from build123d import *

# Parameters (mm, degrees)
EXTRUDE_1_DEPTH     = 50
SKETCH_2_R          = 11.05
CUT_EXTRUDE_1_DEPTH = 88.76388779
CHAMFER_1_SIZE      = 5
SKETCH_3_R          = 1.75
CUT_EXTRUDE_2_DEPTH = 88.76388779
EXTRUDE_3_DEPTH     = 3
EXTRUDE_START       = -3
EXTRUDE_4_DEPTH     = 3
CUT_EXTRUDE_3_DEPTH = 88.832226432


with BuildPart() as part:
    # 草图1 → 凸台-拉伸1 (new body)
    with BuildSketch(Plane(origin=(0, 0, 0), x_dir=(0, 0, -1), z_dir=(1, 0, 0))):
        Polygon((0, 0), (3, 0), (3, -48.5), (53.5, -48.5), (53.5, -51.5), (0, -51.5), align=None)
    extrude(amount=EXTRUDE_1_DEPTH)

    # 草图2 → 切除-拉伸1 (cut, through all)
    with BuildSketch(Plane(origin=(0, 0, -3), x_dir=(-1, 0, 0), z_dir=(0, 0, -1))):
        with Locations(Location((-25, -21, 0), (0, 0, 90))):
            Circle(SKETCH_2_R)
    extrude(amount=-CUT_EXTRUDE_1_DEPTH, mode=Mode.SUBTRACT)

    # 倒角1
    chamfer_1_edges = [part.edges().sort_by_distance(p)[0] for p in [
        (50, -50, -53.5),
        (50, 0, -1.5),
        (0, 0, -1.5),
        (0, -50, -53.5),
    ]]
    chamfer(chamfer_1_edges, length=CHAMFER_1_SIZE)

    # 草图3 → 切除-拉伸2 (cut, through all)
    with BuildSketch(Plane(origin=(0, 0, -3), x_dir=(-1, 0, 0), z_dir=(0, 0, -1))):
        with Locations(Location((-40.5, -5.5, 0), (0, 0, 90))):
            Circle(SKETCH_3_R)
        with Locations(Location((-9.5, -5.5, 0), (0, 0, 90))):
            Circle(SKETCH_3_R)
        with Locations(Location((-9.5, -36.5, 0), (0, 0, 90))):
            Circle(SKETCH_3_R)
        with Locations(Location((-40.5, -36.5, 0), (0, 0, 90))):
            Circle(SKETCH_3_R)
    extrude(amount=-CUT_EXTRUDE_2_DEPTH, mode=Mode.SUBTRACT)

    # 草图4 → 凸台-拉伸3 (add)
    with BuildSketch(Plane(origin=(50, 0, 0), x_dir=(0, 0, -1), z_dir=(1, 0, 0))):
        with BuildLine():
            Line((3, -28.5), (16, -48.5))
            Line((16, -48.5), (5, -48.5))
            ThreePointArc((5, -48.5), (3.585786438, -47.914213562), (3, -46.5))
            Line((3, -46.5), (3, -28.5))
        make_face()
    extrude(amount=-EXTRUDE_3_DEPTH)

    # 草图5 → 凸台-拉伸4 (add)
    with BuildSketch(Plane.ZY.offset(EXTRUDE_START)):
        with BuildLine():
            Line((-5, -48.5), (-16, -48.5))
            Line((-16, -48.5), (-3, -28.5))
            Line((-3, -28.5), (-3, -46.5))
            ThreePointArc((-3, -46.5), (-3.585786438, -47.914213562), (-5, -48.5))
        make_face()
    extrude(amount=EXTRUDE_4_DEPTH)

    # 草图6 → 切除-拉伸3 (cut, through all)
    with BuildSketch(Plane(origin=(0, -48.5, 0), x_dir=(1, 0, 0), z_dir=(0, 1, 0))):
        with BuildLine():
            Line((12.1, 42.5), (12.1, 12.5))
            ThreePointArc((12.1, 12.5), (10, 10.4), (7.9, 12.5))
            Line((7.9, 12.5), (7.9, 42.5))
            ThreePointArc((7.9, 42.5), (10, 44.6), (12.1, 42.5))
        make_face()
        with BuildLine():
            Line((42.1, 42.5), (42.1, 12.5))
            ThreePointArc((42.1, 12.5), (40, 10.4), (37.9, 12.5))
            Line((37.9, 12.5), (37.9, 42.5))
            ThreePointArc((37.9, 42.5), (40, 44.6), (42.1, 42.5))
        make_face()
    extrude(amount=-CUT_EXTRUDE_3_DEPTH, mode=Mode.SUBTRACT)


solid = part.part
Could you check a few things on this model? Use its own coordinates, in mm. A direction names the side the tool comes from. Coordinates: 2 decimals unless noted, no trailing zeros. Order: outer loops, then holes, each group sorted by start corner. A loop starts at its lowest first (then second) coordinate and runs counter-clockwise, first axis right, second up.
Q1. Suppose I cut it at C-C on x = 32. Please give me the cut outline in (y, z), and give its area (3 significant figures).
Q2. Suppose I cut it at B-B on y = -36.5. Please give me the cut outline in (x, z), and give its area (3 significant figures).
Q3. Please list where these lines run through material, in increasing order: L1, parallel to X at y = -36.5, z = -7; L2, parallel to X at y = -36.5, z = -1.95; L3, parallel to X at y = -21, z = -2.3.
Q4. Suppose I cut it at D-D on x = 9.5. Please give me the cut outline in (y, z), and give its area (3 significant figures).
Q5. Thinking about a two-plate mould opening in Z: for faces 1 (the cylindrical face through (11, -35.6, -1.5)), 2 (the flat face through (1.52, -38.64, -9.59)), 3 (the cylindrical face through (10, -50, -44.6)), 4 (the cylindrical face through (40, -50, -44.6)), which applies, released by +Z, released by -Z, zero draft, split by the parting line, or undercut?
Q6. Suppose I cut it at A-A on z = -35.5. Please give me the cut outline in (x, y).
Q7. Which directions (+Z, -Z, +X, -X, +Y, -Y) give clear straight access to the entire face, cutting with the end or side of a thin tool? Please do faces 5 (the flat face through (48.52, -38.36, -9.41)), 6 (the flat face through (37.9, -50, -27)), 7 (the flat face through (3, -43, -7)).
Q8. Will these pins go through, and if not, where does the flat tip stop? pin 1 (8 mm diameter, centred on x = 43, z = -38.5, fed in from +Y); pin 2 (5.5 mm diameter, centred on x = 40.5, y = -36.5, fed in from -Z).
Answer:
1. outline: (-51.5, -53.5) - (-48.5, -53.5) - (-48.5, -3) - (-29.55, -3) - (-29.55, 0) - (-51.5, 0) - close; (-12.45, -3) - (0, -3) - (0, 0) - (-12.45, 0) - close
1. area: 255 mm2
2. outline: (0, -8.2) - (3, -8.2) - (3, -3) - (7.75, -3) - (7.75, 0) - (0, 0) - close; (11.25, -3) - (38.75, -3) - (38.75, 0) - (11.25, 0) - close; (42.25, -3) - (47, -3) - (47, -8.2) - (50, -8.2) - (50, 0) - (42.25, 0) - close
2. area: 160 mm2
3. L1: x = 0 to 3, 47 to 50
3. L2: x = 0 to 7.75, 11.25 to 38.75, 42.25 to 50
3. L3: x = 0 to 13.95, 36.05 to 50
4. outline: (-51.5, -53.5) - (-48.5, -53.5) - (-48.5, -44.54) - (-51.5, -44.54) - close; (-51.5, -10.46) - (-48.5, -10.46) - (-48.5, -3) - (-38.25, -3) - (-38.25, 0) - (-51.5, 0) - close; (-34.75, -3) - (-7.25, -3) - (-7.25, 0) - (-34.75, 0) - close; (-3.75, -3) - (0, -3) - (0, 0) - (-3.75, 0) - close
4. area: 183 mm2
5. face 1: zero draft
5. face 2: released by -Z
5. face 3: undercut
5. face 4: undercut
6. outline: (0, -51.5) - (7.9, -51.5) - (7.9, -48.5) - (0, -48.5) - close; (12.1, -51.5) - (37.9, -51.5) - (37.9, -48.5) - (12.1, -48.5) - close; (42.1, -51.5) - (50, -51.5) - (50, -48.5) - (42.1, -48.5) - close
7. face 5: -Z, +X, -X, +Y
7. face 6: +Y, -Y
7. face 7: -Z, +Y
8. pin 1: stops at y = -48.5
8. pin 2: stops at z = -3
